```python
from build123d import *

# Parameters (mm, degrees)
SKETCH_1_W          = 8
SKETCH_1_H          = 13.5
EXTRUDE_1_DEPTH     = 2
EXTRUDE_2_DEPTH     = 2
SKETCH_3_W          = 1
SKETCH_3_H          = 9.5
EXTRUDE_3_DEPTH     = 2
CUT_EXTRUDE_1_REACH = 22.791
CUT_EXTRUDE_2_REACH = 21.397
FILLET_1_R          = 1


with BuildPart() as part:
    # 草图1 → 凸台-拉伸1 (new body)
    with BuildSketch(Plane.XY):
        with Locations((0, 6.75)):
            Rectangle(SKETCH_1_W, SKETCH_1_H)
    extrude(amount=EXTRUDE_1_DEPTH)

    # 草图2 → 凸台-拉伸2 (add)
    with BuildSketch(Plane(origin=(0, 0, 0), x_dir=(-1, 0, 0), z_dir=(0, -1, 0))):
        Polygon((-4, -2), (-5, -2), (-5, -15), (5, -15), (5, -2), (4, -2), (4, 0), (-4, 0), align=None)
    extrude(amount=-EXTRUDE_2_DEPTH)

    # 草图3 → 凸台-拉伸3 (add)
    with BuildSketch(Plane(origin=(0, 0, 0), x_dir=(-1, 0, 0), z_dir=(0, -1, 0))):
        with Locations((4.5, -6.75)):
            Rectangle(SKETCH_3_W, SKETCH_3_H)
        with Locations((-4.5, -6.75)):
            Rectangle(SKETCH_3_W, SKETCH_3_H)
    extrude(amount=EXTRUDE_3_DEPTH)

    # 草图4 → 切除-拉伸1 (cut, up to next)
    with BuildSketch(Plane(origin=(0, 0, 0), x_dir=(-1, 0, 0), z_dir=(0, -1, 0)), mode=Mode.PRIVATE) as cut_extrude_1_sk1:
        with BuildLine():
            Line((1.5, -8.822875656), (1.5, -10.75))
            Line((1.5, -10.75), (-1.5, -10.75))
            Line((-1.5, -10.75), (-1.5, -8.822875656))
            ThreePointArc((-1.5, -8.822875656), (-2, -7.5), (-1.5, -6.177124344))
            Line((-1.5, -6.177124344), (-1.5, -4.25))
            Line((-1.5, -4.25), (1.5, -4.25))
            Line((1.5, -4.25), (1.5, -6.177124344))
            ThreePointArc((1.5, -6.177124344), (2, -7.5), (1.5, -8.822875656))
        make_face()
    cut_extrude_1_tool1 = extrude(cut_extrude_1_sk1.sketch, amount=-CUT_EXTRUDE_1_REACH, mode=Mode.PRIVATE) & part.part
    add(cut_extrude_1_tool1.solids().sort_by_distance((0, 0, 7.5))[0], mode=Mode.SUBTRACT)

    # 草图5 → 切除-拉伸2 (cut, up to next)
    with BuildSketch(Plane.XY.offset(2), mode=Mode.PRIVATE) as cut_extrude_2_sk1:
        with BuildLine():
            Line((-1.5, 8.572875656), (-1.5, 10.5))
            Line((-1.5, 10.5), (1.5, 10.5))
            Line((1.5, 10.5), (1.5, 8.572875656))
            ThreePointArc((1.5, 8.572875656), (2, 7.25), (1.5, 5.927124344))
            Line((1.5, 5.927124344), (1.5, 4))
            Line((1.5, 4), (-1.5, 4))
            Line((-1.5, 4), (-1.5, 5.927124344))
            ThreePointArc((-1.5, 5.927124344), (-2, 7.25), (-1.5, 8.572875656))
        make_face()
    cut_extrude_2_tool1 = extrude(cut_extrude_2_sk1.sketch, amount=-CUT_EXTRUDE_2_REACH, mode=Mode.PRIVATE) & part.part
    add(cut_extrude_2_tool1.solids().sort_by_distance((0, 7.25, 2))[0], mode=Mode.SUBTRACT)

    # 圆角1
    fillet_1_edges = [part.edges().sort_by_distance(p)[0] for p in [
        (-5, 1, 15),
        (5, 1, 15),
        (-4, 13.5, 1),
        (4, 13.5, 1),
    ]]
    fillet(fillet_1_edges, radius=FILLET_1_R)


solid = part.part
```
Input: part model. Units: mm. Frame: model coordinates. A direction names the side the tool comes from. Give positions to 0.01 mm unless a question says otherwise; leave off trailing zeros. Loops run counter-clockwise (first coordinate to the right, second up) from the corner with the lowest first, then second, coordinate; pieces in that order, holes last.
1) Contact query for flat-ended pins moving along their axis: pin 1 (2 mm diameter, centred on y = 9, z = 1, fed in from +X); pin 2 (1.5 mm diameter, centred on x = -0.5, z = 3, fed in from -Y); pin 3 (4 mm diameter, centred on x = 0, y = 10.5, fed in from +Z). Output: stop coordinate, or through.
A:
pin 1: stops at x = 4
pin 2: stops at y = 0
pin 3: stops at z = 2
2) Section query C-C on z = 4. Return the cut outline in (x, y).
A:
outline: (-5, -2) - (-4, -2) - (-4, 0) - (4, 0) - (4, -2) - (5, -2) - (5, 2) - (-5, 2) - close
3) Section query D-D on x = -2.5. Return the cut outline in (y, z), and give its area (3 significant figures).
A:
outline: (0, 0) - (13.5, 0) - (13.5, 2) - (2, 2) - (2, 15) - (0, 15) - close
area: 53.0 mm2
4) Reachability of faces 1 (the flat face through (0, 10.5, 1)), 2 (the flat face through (-1.5, 1, 5)), 3 (the flat face through (-4.5, -1, 11.5)), 4 (the flat face through (-4, 6, 1)) from +Z, -Z, +X, -X, +Y, -Y: full face, straight path, thin tool, end or side. Return the list, or none.
A:
face 1: +Z, -Z
face 2: +Y, -Y
face 3: +Z, +X, -X, -Y
face 4: -Z, -X, +Y, -Y
5) Mould query, pull axis Z, two halves, no side actions, for faces 5 (the flat face through (0, 4, 1)), 6 (the flat face through (0, 1, 4.25)), 7 (the flat face through (0, 1, 10.75)), 8 (the flat face through (4.5, -1, 11.5)). Classes: released by +Z, released by -Z, zero draft, split by the parting line, or undercut.
A:
face 5: zero draft
face 6: undercut
face 7: undercut
face 8: released by +Z
6) Section query A-A on x = 0.25. Return the cut outline in (y, z), and give its area (3 significant figures).
A:
outline: (0, 0) - (4, 0) - (4, 2) - (2, 2) - (2, 4.25) - (0, 4.25) - close; (0, 10.75) - (2, 10.75) - (2, 15) - (0, 15) - close; (10.5, 0) - (13.5, 0) - (13.5, 2) - (10.5, 2) - close
area: 27.0 mm2
7) Line query: L1, parallel to Z at x = -0.5, y = 10.75; L2, parallel to Z at x = -1, y = 0.25. Output: solid intervals per line, ascending.
A:
L1: z = 0 to 2
L2: z = 0 to 4.25, 10.75 to 15
8) Section query B-B on z = 7. Return the cut outline in (x, y).
A:
outline: (-5, -2) - (-4, -2) - (-4, 0) - (-1.94, 0) - (-1.94, 2) - (-5, 2) - close; (1.94, 0) - (4, 0) - (4, -2) - (5, -2) - (5, 2) - (1.94, 2) - close
